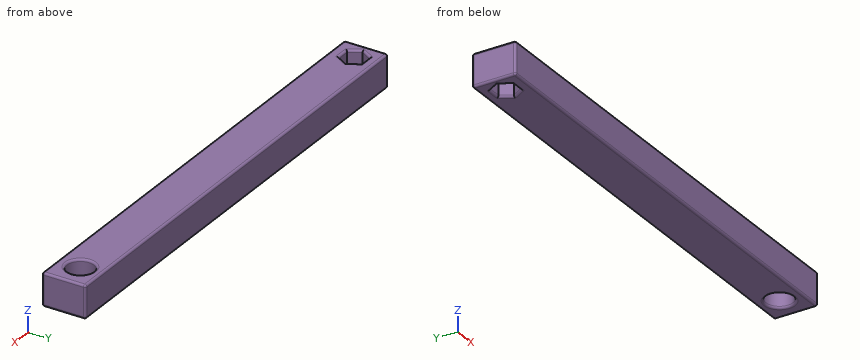
```python
from build123d import *

# Parameters (mm, degrees)
SKETCH1_W           = 558.8
SKETCH1_H           = 50.8
SKETCH1_R           = 15.661500759
BOSS_EXTRUDE1_DEPTH = 38.354
FILLET2_R           = 2.54
FILLET3_R           = 2.54
FILLET4_R           = 2.54
FILLET5_R           = 2.54
FILLET6_R           = 2.54
FILLET7_R           = 2.54
FILLET8_R           = 2.54
FILLET9_R           = 2.54


with BuildPart() as part:
    # Sketch1 → Boss-Extrude1 (new body)
    with BuildSketch(Plane.XY):
        with Locations((250.222913627, 20.811022444)):
            Rectangle(SKETCH1_W, SKETCH1_H)
        with Locations((499.940155303, 21.505918387)):
            Circle(SKETCH1_R, mode=Mode.SUBTRACT)
        Polygon((9.266544067, 21.505918387), (1.58198055, 34.815972833), (-13.787146484, 34.815972833), (-21.471710001, 21.505918387), (-13.787146484, 8.195863942), (1.58198055, 8.195863942), align=None, mode=Mode.SUBTRACT)
    extrude(amount=BOSS_EXTRUDE1_DEPTH)

    # Fillet2
    fillet2_edges = [part.edges().sort_by_distance(p)[0] for p in [
        (-29.177086373, 46.211022444, 19.177),
    ]]
    fillet(fillet2_edges, radius=FILLET2_R)

    # Fillet3
    fillet3_edges = [part.edges().sort_by_distance(p)[0] for p in [
        (251.492913627, 46.211022444, 38.354),
        (-29.177086373, 19.541022444, 38.354),
        (-28.433137597, 45.467073669, 38.354),
    ]]
    fillet(fillet3_edges, radius=FILLET3_R)

    # Fillet4
    fillet4_edges = [part.edges().sort_by_distance(p)[0] for p in [
        (-29.177086373, 19.541022444, 0),
        (-28.433137597, 45.467073669, 0),
        (251.492913627, 46.211022444, 0),
    ]]
    fillet(fillet4_edges, radius=FILLET4_R)

    # Fillet5
    fillet5_edges = [part.edges().sort_by_distance(p)[0] for p in [
        (529.622913627, 19.541022444, 38.354),
        (529.622913627, 46.211022444, 19.177),
        (529.622913627, 45.467073669, 37.610051224),
        (529.622913627, 19.541022444, 0),
        (529.622913627, 45.467073669, 0.743948776),
    ]]
    fillet(fillet5_edges, radius=FILLET5_R)

    # Fillet6
    fillet6_edges = [part.edges().sort_by_distance(p)[0] for p in [
        (250.222913627, -4.588977556, 38.354),
        (-29.177086373, -4.588977556, 19.177),
        (-28.433137597, -4.588977556, 37.610051224),
        (250.222913627, -4.588977556, 0),
        (-28.433137597, -4.588977556, 0.743948776),
        (529.622913627, -4.588977556, 19.177),
        (528.878964852, -4.588977556, 37.610051224),
        (528.878964852, -4.588977556, 0.743948776),
    ]]
    fillet(fillet6_edges, radius=FILLET6_R)

    # Fillet7
    fillet7_edges = [part.edges().sort_by_distance(p)[0] for p in [
        (484.278654543, 21.505918387, 0),
        (484.278654543, 21.505918387, 38.354),
    ]]
    fillet(fillet7_edges, radius=FILLET7_R)

    # Fillet8
    fillet8_edges = [part.edges().sort_by_distance(p)[0] for p in [
        (5.424262309, 14.850891165, 0),
        (5.424262309, 28.16094561, 0),
        (-6.102582967, 34.815972833, 0),
        (-17.629428242, 28.16094561, 0),
        (-17.629428242, 14.850891165, 0),
        (-6.102582967, 8.195863942, 0),
    ]]
    fillet(fillet8_edges, radius=FILLET8_R)

    # Fillet9
    fillet9_edges = [part.edges().sort_by_distance(p)[0] for p in [
        (5.424262309, 14.850891165, 38.354),
        (5.424262309, 28.16094561, 38.354),
        (-6.102582967, 34.815972833, 38.354),
        (-17.629428242, 28.16094561, 38.354),
        (-17.629428242, 14.850891165, 38.354),
        (-6.102582967, 8.195863942, 38.354),
    ]]
    fillet(fillet9_edges, radius=FILLET9_R)


solid = part.part
```
The model under review builds one solid part; all positions refer to its coordinate system, in mm. Round coordinates to 2 decimals unless told otherwise and drop trailing zeros. Order: outer loops, then holes, each group sorted by start corner. A loop starts at its lowest first (then second) coordinate and runs counter-clockwise, first axis right, second up. Notation, with made-up numbers: (89.5, 45.25) -> (148.5, 45.25) arc R21 cw to (148.5, 84.25) -> close; hole circle Ø6 at (32, 38.5). An arc over 180 degrees is marked (long way). One line per item, written item: value. Start each with the question number.
Q1. Take a section at B-B (y = 27). Count the separate pieces of the cut face and the enclosed holes in it, and give its area (3 significant figures).
Q2. Take a section at A-A (z = 10.5). Write out the cut boundary in (x, y), and give its area (3 significant figures).
Q3. Wall thickness on line 1 (X direction, y = 21.5, z = 34.5); line 2 (X direction, y = 11.5, z = 14); line 3 (X direction, y = 7.5, z = 4.5): over which ranges is each line inside the solid? List them lowest first.
Reported:
1. separate pieces: 3
1. enclosed holes: 0
1. area: 19,400 mm2
2. outline: (-29.18, -2.05) arc R2.54 ccw to (-26.64, -4.59) -> (527.08, -4.59) arc R2.54 ccw to (529.62, -2.05) -> (529.62, 43.67) arc R2.54 ccw to (527.08, 46.21) -> (-26.64, 46.21) arc R2.54 ccw to (-29.18, 43.67) -> close; hole (-21.47, 21.51) -> (-13.79, 8.2) -> (1.58, 8.2) -> (9.27, 21.51) -> (1.58, 34.82) -> (-13.79, 34.82) -> close; hole circle Ø31.32 at (499.94, 21.51)
2. area: 27,000 mm2
3. line 1: x = -29.18 to -21.47, 9.26 to 484.28, 515.6 to 529.62
3. line 2: x = -29.18 to -15.69, 3.49 to 487.89, 511.99 to 529.62
3. line 3: x = -29.18 to 492.93, 506.95 to 529.62
